```python
from build123d import *

# Parameters (mm, degrees)
F1_W     = 156.05
F1_H     = 66.675
F2_DEPTH = 50
F3_D     = 5.6
F3_DEPTH = 20
F3_TIP   = 1.6824097333
F4_W     = 119.824
F4_H     = 62.675
F5_DEPTH = 45
F6_W     = 40
F6_H     = 5
F7_DEPTH = 66.676
F9_D     = 4


with BuildPart() as f2:
    # F1 (on Front) → F2 (new body)
    with BuildSketch(Plane.XZ):
        Rectangle(F1_W, F1_H)
    extrude(amount=-F2_DEPTH)

    # F3
    with Locations(Plane.XZ):
        with Locations((-68.262, 19.0495), (-68.262, -19.0495), (68.262, -19.0495), (68.262, 19.0495)):
            Hole(F3_D / 2, depth=F3_DEPTH)
            with Locations((0, 0, -(F3_DEPTH + F3_TIP / 2))):  # 118° drill point
                Cone(0, F3_D / 2, F3_TIP, mode=Mode.SUBTRACT)

    # F4 (on face) → F5 (cut)
    with BuildSketch(Plane.XZ):
        Rectangle(F4_W, F4_H)
    extrude(amount=-F5_DEPTH, mode=Mode.SUBTRACT)

    # F6 (on face) → F7 (cut, through all)
    with BuildSketch(Plane(origin=(0, 0, -33.3375), x_dir=(1, 0, 0), z_dir=(0, 0, -1))):
        with Locations((0, -42.5)):
            Rectangle(F6_W, F6_H)
    extrude(amount=-F7_DEPTH, mode=Mode.SUBTRACT)

    # F9 (through all)
    with Locations(Plane(origin=(0, 0, -33.3375), x_dir=(1, 0, 0), z_dir=(0, 0, -1))):
        with Locations((-49.912, -25), (49.912, -25)):
            Hole(F9_D / 2)


solid = f2.part
```
For this review, take the finished solid that the model builds, in its own axes (mm). A direction names the side the tool comes from. Give positions to 0.01 mm unless a question says otherwise; leave off trailing zeros. Write each loop counter-clockwise with the first axis right and the second up, starting at its lowest first coordinate (ties: lowest second). Pieces come first, ordered by that corner, then holes.
Item 1: Insertion check: P1, Ø5, axis at x = -68.26, z = -19.05, coming from the -Y side; P2, Ø3.5, axis at x = 68.26, z = 19.05, coming from the -Y side. Each pin has a flat end and moves straight along its axis. Give the tip position at first contact, or say it passes through.
Item 2: Take a section at C-C (z = 12.5). Give the boundary of the cut face in (x, y) (3 decimals).
Item 3: Take a section at B-B (y = 25). Give the boundary of the cut face in (x, z) (1 decimal).
Item 4: The part is to be moulded in two halves that separate along X. For faces 3 (the face through (-1, 50, 0)), 4 (the face through (-1, 45, 0)), 5 (the face through (-78.025, 25, 0)), say which applies: +X half, -X half, draft (parallel to the pull), parting line (faces both ways), or undercut.
Item 5: Machinability: for faces 1 (the face through (-70.85, 10.14, 17.98)), 2 (the face through (78.025, 25, 0)), which of the approach directions +Z, -Z, +X, -X, +Y, -Y give a long, thin tool a straight path to every point of the face, cutting with its end or side? Answer none if there is none.
Item 6: Take a section at A-A (x = -12.5). Give the boundary of the cut face in (y, z), and give its area (3 significant figures).
Item 7: Wall thickness on probe 1 along X at (y, z) = (25, -32.8) (3 decimals); probe 2 along Y at (x, z) = (-11.5, 31.5); probe 3 along Z at (x, y) = (37, 42.5): over which ranges is each line inside the solid? List them lowest first.
Item 8: Take a section at D-D (y = 15.5). Give the boundary of the cut face in (x, z) (1 decimal).
Established:
1. P1: stops at y = 20.18
1. P2: stops at y = 20.63
2. outline: (-78.025, 0) - (-59.912, 0) - (-59.912, 45) - (59.912, 45) - (59.912, 0) - (78.025, 0) - (78.025, 50) - (-78.025, 50) - close
3. outline: (-78, -33.3) - (-51.9, -33.3) - (-51.9, -31.3) - (-59.9, -31.3) - (-59.9, 31.3) - (-51.9, 31.3) - (-51.9, 33.3) - (-78, 33.3) - close; (-47.9, -33.3) - (47.9, -33.3) - (47.9, -31.3) - (-47.9, -31.3) - close; (-47.9, 31.3) - (47.9, 31.3) - (47.9, 33.3) - (-47.9, 33.3) - close; (51.9, -33.3) - (78, -33.3) - (78, 33.3) - (51.9, 33.3) - (51.9, 31.3) - (59.9, 31.3) - (59.9, -31.3) - (51.9, -31.3) - close
4. face 3: draft
4. face 4: undercut
4. face 5: -X half
5. face 1: -Y
5. face 2: +Z, -Z, +X, +Y, -Y
6. outline: (0, -33.34) - (40, -33.34) - (40, -31.34) - (0, -31.34) - close; (0, 31.34) - (40, 31.34) - (40, 33.34) - (0, 33.34) - close; (45, -33.34) - (50, -33.34) - (50, 33.34) - (45, 33.34) - close
6. area: 493 mm2
7. probe 1: x = -78.025 to -51.912, -47.912 to 47.912, 51.912 to 78.025
7. probe 2: y = 0 to 40, 45 to 50
7. probe 3: z = -33.34 to -31.34, 31.34 to 33.34
8. outline: (-78, -33.3) - (78, -33.3) - (78, 33.3) - (-78, 33.3) - close; hole circle Ø5.6 at (-68.3, -19); hole circle Ø5.6 at (-68.3, 19); hole (-59.9, -31.3) - (59.9, -31.3) - (59.9, 31.3) - (-59.9, 31.3) - close; hole circle Ø5.6 at (68.3, -19); hole circle Ø5.6 at (68.3, 19)
